Input: part model. Units: mm. Frame: model coordinates. A direction names the side the tool comes from. Coordinates: 2 decimals unless noted, no trailing zeros. Loops run counter-clockwise (first coordinate to the right, second up) from the corner with the lowest first, then second, coordinate; pieces in that order, holes last. Notation, with made-up numbers: (85, -4.75) - (117, -4.75) arc R6 cw to (117, 1.25) - close; hole circle Ø2 at (74.25, 87.25). An arc over 180 degrees is marked (long way). Use one line per item in the form item = value.
Autodesk Inventor part; units mm, degrees
ref_plane "YZ Plane" through (0, 0, 0) normal (1, 0, 0) x (0, 1, 0)
ref_plane "XZ Plane" through (0, 0, 0) normal (0, 1, 0) x (-1, 0, 0)
ref_plane "XY Plane" through (0, 0, 0) normal (0, 0, 1) x (1, 0, 0)
sketch "Sketch2" plane through (0, 0, 0) normal (0, 0, 1) x (1, 0, 0)
  circle A0 centre (0, 0) radius 22.25
  dimension "d2" = 44.5
extrude "Extrusion1" add sketch "Sketch2" along normal blind 83
sketch "Sketch9" plane through (0, 0, 83) normal (0, 0, 1) x (1, 0, 0)
  circle A0 centre (0, 0) radius 22.25
  line L0 (-31.15, 0) -> (31.15, 0)
  line L1 (0, -31.15) -> (0, 31.15)
  circle A1 centre (0, 0) radius 20.25
  dimension "d54" = 40.5
extrude "Extrusion7" cut sketch "Sketch9" against normal blind 82.7 contours A1 L1 L0 | L0 L1 A1 | L1 L0 A1 | A1 L0 L1
fillet "Fillet12" radius 17 1 edges at (-20.25, 0, 0.3)
sketch "Sketch18" plane through (0, 0, 0.3) normal (0, 0, 1) x (1, 0, 0)
  line L0 (-31.15, 0) -> (31.15, 0)
  line L1 (0, -31.15) -> (0, 31.15)
  line L2 (1.55, 2.35) -> (-1.55, 2.35)
  line L3 (-1.55, 2.35) -> (-1.55, -2.35)
  line L4 (-1.55, -2.35) -> (1.55, -2.35)
  line L5 (1.55, -2.35) -> (1.55, 2.35)
  line L6 (1.55, 2.35) -> (-1.55, -2.35) construction
  line L7 (-1.55, 2.35) -> (1.55, -2.35) construction
  point P0 (0, 0)
  dimension "d122" = 3.1
  dimension "d123" = 4.7
extrude "Extrusion15" cut sketch "Sketch18" against normal through all
chamfer "Chamfer9" distance 4 angle 45 1 edges at (-22.25, 0, 0)
equation "\"BendRadius\" = Thickness"
equation "\"BendReliefWidth\" = Thickness"
equation "\"BendReliefDepth\" = 0.5 * Thickness"
equation "\"CornerReliefSize\" = 4 * Thickness"
equation "\"MinimumRemnant\" = 2 * Thickness"
equation "\"TransitionRadius\" = BendRadius"
equation "\"JacobiRadiusSize\" = BendRadius"
equation "\"GapSize\" = Thickness"
properties part number "_3DPrint"
Q1. Cut plane A-A, the plane z = 48. Return loops of the section in (x, y), then the cut area to 3 significant figures.
Check values:
outline = circle Ø44.5 at (0, 0); hole circle Ø40.5 at (0, 0)
area = 267 mm²
Q2. Pull-direction query (Y, two-part tool) for faces 1 (the flat face through (5, -20, 83)), 2 (the cylindrical face through (11, 17, 51)), 3 (the conical face through (17.646, 5.557, 0.25)); classes: pulls with the +Y half, pulls with the -Y half, needs draft (parallel to the pull), parting line crosses it, or undercut.
Check values:
face_1 = needs draft
face_2 = undercut
face_3 = parting line crosses it
Q3. First-contact query: P1, Ø12, axis at x = -5, y = 11.5, coming from the -Z side; P2, Ø5, axis at y = -10, z = 8.5, coming from the -X side; P3, Ø24.5, axis at x = 0, y = 0, coming from the +Z side; P4, Ø5, axis at y = 4, z = 37, coming from the -X side. Flat tips, straight axial feed; report the tip coordinate or a pass-through.
Check values:
P1 = 0
P2 = -20.95
P3 = 2.88
P4 = -22.2
Q4. Ray query, line 1 along Y through (x, z) = (0, 61); line 2 along X through (y, z) = (18, 48); line 3 along Y through (x, z) = (-16, 19.5). Return the intervals inside material, ascending. Write a range as [from, to].
Check values:
line_1 = [-22.25, -20.25], [20.25, 22.25]
line_2 = [-13.08, -9.28], [9.28, 13.08]
line_3 = [-15.46, -12.41], [12.41, 15.46]
Q5. Set-up query: faces 4 (the flat face through (2, 0, 0.3)), 5 (the cylindrical face through (-16.399, -15.038, 42.947)). Return all of +Z, -Z, +X, -X, +Y, -Y with unobstructed straight access to the full face (end or side cutting, diameter ignored); none if empty.
Check values:
face_4 = +Z
face_5 = +Z, -Z
